Input: part model. Units: mm. Frame: model coordinates. Face numbers are marked on the shaded views. A direction names the side the tool comes from. Round coordinates to 2 decimals unless told otherwise and drop trailing zeros. Loops run counter-clockwise (first coordinate to the right, second up) from the corner with the lowest first, then second, coordinate; pieces in that order, holes last. Notation, with made-up numbers: M -33,80.25 L -26,80.25 A20 cw -26,93.25 Z; hole C 54,32.5 d10. An arc over 180 degrees is marked long. Put each result on its own line as item: value. Start each with the question number.
1) Section A-A on z = 1.5. Output: boundary loops of the cut face in (x, y), plus the area to 3 significant figures.
2) Line query: probe 1 along X at (y, z) = (-9.5, 6.75); probe 2 along Y at (x, z) = (8.5, 8); probe 3 along Y at (x, z) = (5, 9.25). Output: solid intervals per line, ascending.
3) Reachability of the marked faces 1, 2, 3 and 4 from +Z, -Z, +X, -X, +Y, -Y: full face, straight path, thin tool, end or side. Return the list, or none.
4) Section D-D on x = -18. Output: boundary loops of the cut face in (y, z).
5) Pin query (flat end, axial travel): pin 1 (3 mm diameter, centred on x = 63.5, z = 4.5, fed in from -Y); pin 2 (5 mm diameter, centred on x = 48.5, z = 5, fed in from +Y); pin 3 (5 mm diameter, centred on x = 5.5, z = 2.5, fed in from +Y); pin 4 (12 mm diameter, centred on x = -55.5, y = 13, fed in from -Z). Return the tip coordinate at first contact, or that it passes through.
6) Section B-B on x = 34.5. Output: boundary loops of the cut face in (y, z), plus the area to 3 significant figures.
7) Draft query along X for the marked faces 5, 6 and 7. Return one class per face: +X half, -X half, draft (parallel to the pull), parting line (faces both ways), or undercut.
8) Section C-C on y = 18. Output: boundary loops of the cut face in (x, z), plus the area to 3 significant figures.
from build123d import *

# Parameters (mm, degrees)
SKETCH_1_W          = 140
SKETCH_1_H          = 70
EXTRUDE_2_DEPTH     = 10
SKETCH_2_W          = 10.079720787
SKETCH_2_H          = 10
SKETCH_2_W_2        = 5
SKETCH_2_H_2        = 25
CUT_EXTRUDE_2_DEPTH = 10
FILLET_1_R          = 2


with BuildPart() as part:
    # 草图1 → 凸台-拉伸2 (new body)
    with BuildSketch(Plane.XY):
        Rectangle(SKETCH_1_W, SKETCH_1_H)
    extrude(amount=EXTRUDE_2_DEPTH)

    # 草图2 → 切除-拉伸2 (cut)
    with BuildSketch(Plane.XY.offset(10)):
        Polygon((39.920279213, 22.281959867), (59.920279213, 22.281959867), (70, 22.281959867), (70, 35), (-20, 35), align=None)
        with Locations((64.960139607, 17.281959867)):
            Rectangle(SKETCH_2_W, SKETCH_2_H)
        with Locations((64.960139607, -17.281959867)):
            Rectangle(SKETCH_2_W, SKETCH_2_H)
        Polygon((70, -22.281959867), (59.920279213, -22.281959867), (39.920279213, -22.281959867), (-20, -35), (70, -35), align=None)
        Polygon((40, -12.5), (40, 0), (40, 12.5), (-20, 12.5), (-20, -12.5), align=None)
        with Locations((-22.5, 0)):
            Rectangle(SKETCH_2_W_2, SKETCH_2_H_2)
    extrude(amount=-CUT_EXTRUDE_2_DEPTH, mode=Mode.SUBTRACT)

    # 圆角1
    fillet_1_edges = [part.edges().sort_by_distance(p)[0] for p in [
        (40, -12.5, 5),
        (-25, -12.5, 5),
        (-25, 12.5, 5),
        (40, 12.5, 5),
    ]]
    fillet(fillet_1_edges, radius=FILLET_1_R)


solid = part.part
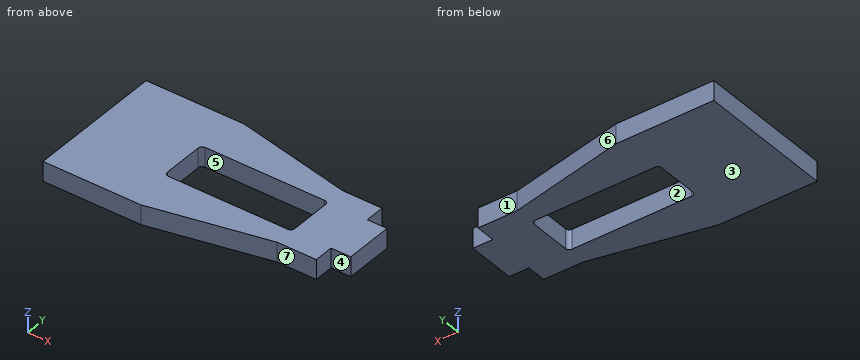
Geometry results:
1. outline: M -70,-35 L -20,-35 L 39.92,-22.28 L 59.92,-22.28 L 59.92,-12.28 L 70,-12.28 L 70,12.28 L 59.92,12.28 L 59.92,22.28 L 39.92,22.28 L -20,35 L -70,35 Z; hole M -25,-10.5 A2 ccw -23,-12.5 L 38,-12.5 A2 ccw 40,-10.5 L 40,10.5 A2 ccw 38,12.5 L -23,12.5 A2 ccw -25,10.5 Z
1. area: 6,450 mm²
2. probe 1: x = -70 to -25, 40 to 70
2. probe 2: y = -28.95 to -12.5, 12.5 to 28.95
2. probe 3: y = -29.69 to -12.5, 12.5 to 29.69
3. face 1: +Z, -Z, +X, +Y
3. face 2: +Z, -Z
3. face 3: -Z, +X, -X, +Y, -Y
3. face 4: +Z, -Z, +X, -Y
4. outline: M -34.58,0 L -12.5,0 L -12.5,10 L -34.58,10 Z; M 12.5,0 L 34.58,0 L 34.58,10 L 12.5,10 Z
5. pin 1: stops at y = -12.28
5. pin 2: stops at y = 22.28
5. pin 3: stops at y = 30.12
5. pin 4: stops at z = 0
6. outline: M -23.43,0 L -12.5,0 L -12.5,10 L -23.43,10 Z; M 12.5,0 L 23.43,0 L 23.43,10 L 12.5,10 Z
6. area: 219 mm²
7. face 5: undercut
7. face 6: +X half
7. face 7: draft
8. outline: M -70,0 L 59.92,0 L 59.92,10 L -70,10 Z
8. area: 1,300 mm²
